Input: part model. Units: mm. Frame: model coordinates. A direction names the side the tool comes from. Coordinates: 2 decimals unless noted, no trailing zeros. Order: outer loops, then holes, each group sorted by start corner. A loop starts at its lowest first (then second) coordinate and runs counter-clockwise, first axis right, second up. Notation, with made-up numbers: (55.5, -23.5) - (75.5, -23.5) arc R37 ccw to (75.5, 12.5) - close; hole circle Ø7 at (-17.5, 52). An arc over 180 degrees is marked (long way). Use a Markdown table: item, result. Add a question column.
from build123d import *

# Parameters (mm, degrees)
F0_W     = 3.1821551265
F0_H     = 16.2380066949
F1_DEPTH = 25.4


with BuildPart() as f1:
    # F0 (on Front) → F1 (new body)
    with BuildSketch(Plane.XZ):
        with BuildLine():
            ThreePointArc((50.8, 12.7), (48.9401280605, 17.1901280605), (44.45, 19.05))
            Line((44.45, 19.05), (-44.45, 19.05))
            ThreePointArc((-44.45, 19.05), (-48.9401280605, 17.1901280605), (-50.8, 12.7))
            Line((-50.8, 12.7), (-50.8, -12.7))
            ThreePointArc((-50.8, -12.7), (-48.9401280605, -17.1901280605), (-44.45, -19.05))
            Line((-44.45, -19.05), (44.45, -19.05))
            ThreePointArc((44.45, -19.05), (48.9401280605, -17.1901280605), (50.8, -12.7))
            Line((50.8, -12.7), (50.8, 12.7))
        make_face()
        with BuildLine():
            Line((-3.4147352544, -7.4699143124), (-8.0493956066, 4.1133974755))
            Line((-8.0493956066, 4.1133974755), (-4.563383065, 4.1133974755))
            Line((-4.563383065, 4.1133974755), (-2.3629211255, -2.4512583259))
            add(Edge.make_bspline(
                [(-2.3629211255, -2.4512583259), (-2.0790982653, -3.3060659989), (-1.9755863987, -4.4747483644)],
                knots=[0, 0, 0, 1, 1, 1], degree=2))
            Line((-1.9755863987, -4.4747483644), (-1.9121436417, -4.4747483644))
            add(Edge.make_bspline(
                [(-1.9121436417, -4.4747483644), (-1.7986144976, -3.3995605882), (-1.4647052503, -2.4512583259)],
                knots=[0, 0, 0, 1, 1, 1], degree=2))
            Line((-1.4647052503, -2.4512583259), (0.6956875795, 4.1133974755))
            Line((0.6956875795, 4.1133974755), (4.1082400867, 4.1133974755))
            Line((4.1082400867, 4.1133974755), (-0.826938588, -9.0459659596))
            add(Edge.make_bspline(
                [(-0.826938588, -9.0459659596), (-1.5081134525, -10.8724495421), (-2.7652817685, -11.7806826947)],
                knots=[0, 0, 0, 1, 1, 1], degree=2))
            add(Edge.make_bspline(
                [(-2.7652817685, -11.7806826947), (-4.0224500844, -12.6889158473), (-5.7020135982, -12.6889158473)],
                knots=[0, 0, 0, 1, 1, 1], degree=2))
            add(Edge.make_bspline(
                [(-5.7020135982, -12.6889158473), (-6.526769439, -12.6889158473), (-7.318134355, -12.5086048538)],
                knots=[0, 0, 0, 1, 1, 1], degree=2))
            Line((-7.318134355, -12.5086048538), (-7.318134355, -9.9842509444))
            add(Edge.make_bspline(
                [(-7.318134355, -9.9842509444), (-6.7438104497, -10.1211537358), (-6.0659746778, -10.1211537358)],
                knots=[0, 0, 0, 1, 1, 1], degree=2))
            add(Edge.make_bspline(
                [(-6.0659746778, -10.1211537358), (-5.2211842822, -10.1211537358), (-4.5900958048, -9.6035944025)],
                knots=[0, 0, 0, 1, 1, 1], degree=2))
            add(Edge.make_bspline(
                [(-4.5900958048, -9.6035944025), (-3.9590073275, -9.0860350692), (-3.6050635254, -8.0442382177)],
                knots=[0, 0, 0, 1, 1, 1], degree=2))
            Line((-3.6050635254, -8.0442382177), (-3.4147352544, -7.4699143124))
        make_face(mode=Mode.SUBTRACT)
        with BuildLine():
            add(Edge.make_bspline(
                [(19.8954692978, -7.5600698092), (18.9471670355, -7.76375445), (17.5781391217, -7.76375445)],
                knots=[0, 0, 0, 1, 1, 1], degree=2))
            add(Edge.make_bspline(
                [(17.5781391217, -7.76375445), (14.7632841672, -7.76375445), (13.1772152426, -6.2077373577)],
                knots=[0, 0, 0, 1, 1, 1], degree=2))
            add(Edge.make_bspline(
                [(13.1772152426, -6.2077373577), (11.5911463181, -4.6517202654), (11.5911463181, -1.8034743862)],
                knots=[0, 0, 0, 1, 1, 1], degree=2))
            add(Edge.make_bspline(
                [(11.5911463181, -1.8034743862), (11.5911463181, 1.1282488049), (13.0570079136, 2.7293436456)],
                knots=[0, 0, 0, 1, 1, 1], degree=2))
            add(Edge.make_bspline(
                [(13.0570079136, 2.7293436456), (14.5228695092, 4.3304384862), (17.1106661755, 4.3304384862)],
                knots=[0, 0, 0, 1, 1, 1], degree=2))
            add(Edge.make_bspline(
                [(17.1106661755, 4.3304384862), (19.5815946054, 4.3304384862), (20.9589702504, 2.923011009)],
                knots=[0, 0, 0, 1, 1, 1], degree=2))
            add(Edge.make_bspline(
                [(20.9589702504, 2.923011009), (22.3363458954, 1.5155835317), (22.3363458954, -0.968701268)],
                knots=[0, 0, 0, 1, 1, 1], degree=2))
            Line((22.3363458954, -0.968701268), (22.3363458954, -2.5147010829))
            Line((22.3363458954, -2.5147010829), (14.8133705543, -2.5147010829))
            add(Edge.make_bspline(
                [(14.8133705543, -2.5147010829), (14.8667960339, -3.8703726268), (15.6180918402, -4.6316857106)],
                knots=[0, 0, 0, 1, 1, 1], degree=2))
            add(Edge.make_bspline(
                [(15.6180918402, -4.6316857106), (16.3693876466, -5.3929987944), (17.7250591905, -5.3929987944)],
                knots=[0, 0, 0, 1, 1, 1], degree=2))
            add(Edge.make_bspline(
                [(17.7250591905, -5.3929987944), (18.7802124119, -5.3929987944), (19.7184973968, -5.1742882374)],
                knots=[0, 0, 0, 1, 1, 1], degree=2))
            add(Edge.make_bspline(
                [(19.7184973968, -5.1742882374), (20.6567823816, -4.9555776804), (21.6785446783, -4.4747483644)],
                knots=[0, 0, 0, 1, 1, 1], degree=2))
            Line((21.6785446783, -4.4747483644), (21.6785446783, -6.9389986093))
            add(Edge.make_bspline(
                [(21.6785446783, -6.9389986093), (20.8437715601, -7.3563851684), (19.8954692978, -7.5600698092)],
                knots=[0, 0, 0, 1, 1, 1], degree=2))
        make_face(mode=Mode.SUBTRACT)
        Polygon((-13.4119781178, 0.9512769038), (-8.0493956066, -7.5533916242), (-11.7223973266, -7.5533916242), (-15.7192910165, -1.1256386142), (-17.0849798378, -2.1073318012), (-17.0849798378, -7.5533916242), (-20.3205604439, -7.5533916242), (-20.3205604439, 7.7029218837), (-17.0849798378, 7.7029218837), (-17.0849798378, 0.7208795232), (-15.8127856057, 2.5173112736), (-11.6789891244, 7.7029218837), (-8.0894647162, 7.7029218837), align=None, mode=Mode.SUBTRACT)
        with Locations((7.3688638863, 0.5656117232)):
            Rectangle(F0_W, F0_H, mode=Mode.SUBTRACT)
    extrude(amount=F1_DEPTH)


solid = f1.part
1) Cut plane B-B (x = 2). Return the cut outline in (y, z).
2) Cut plane A-A (x = -9.5). Return the cut outline in (y, z).
3) Reachability of faces 1 (the flat face through (1.675, -12.522, -2.374)), 2 (the flat face through (-50.8, -13, 0)) from +Z, -Z, +X, -X, +Y, -Y: full face, straight path, thin tool, end or side. Return the list, or none.
4) Cut plane C-C (y = -7). State how many separate pieces and enclosed holes the cut face has, and give its area (3 significant figures).
5) Pull-direction query (Z, two-part tool) for faces 3 (the flat face through (-13.775, -12.522, 5.074)), 4 (the cylindrical face through (-48.89, -12.52, 17.24)), 5 (the cylindrical face through (-48.99, -12.52, -17.14)); classes: pulls with the +Z half, pulls with the -Z half, needs draft (parallel to the pull), parting line crosses it, or undercut.
6) Material intervals for L1, parallel to X at y = -14, z = 0; L2, parallel to Z at x = -20, y = -10; L3, parallel to Z at x = -11.5, y = -7, sorted ascending.
Computed:
| question | item | result |
|---|---|---|
| 1 | outline | (-25.4, -19.05) - (0, -19.05) - (0, -1.51) - (-25.4, -1.51) - close; (-25.4, 4.11) - (0, 4.11) - (0, 19.05) - (-25.4, 19.05) - close |
| 2 | outline | (-25.4, -19.05) - (0, -19.05) - (0, -7.55) - (-25.4, -7.55) - close; (-25.4, -5.25) - (0, -5.25) - (0, 5.91) - (-25.4, 5.91) - close; (-25.4, 7.7) - (0, 7.7) - (0, 19.05) - (-25.4, 19.05) - close |
| 3 | face 1 | +Y, -Y |
| 3 | face 2 | +Z, -Z, -X, +Y, -Y |
| 4 | separate pieces | 1 |
| 4 | enclosed holes | 4 |
| 4 | area | 3,500 mm2 |
| 5 | face 3 | undercut |
| 5 | face 4 | pulls with the +Z half |
| 5 | face 5 | pulls with the -Z half |
| 6 | L1 | x = -50.8 to -20.32, -12.81 to -6.4, -3.18 to -0.66, 2.57 to 5.78, 8.96 to 11.75, 22.28 to 50.8 |
| 6 | L2 | z = -19.05 to -7.55, 7.7 to 19.05 |
| 6 | L3 | z = -19.05 to -7.55, -2.08 to 3.38, 7.7 to 19.05 |
